from build123d import *

# Parameters (mm, degrees)
PAD010_DEPTH = 31
FILLET004_R  = 1.5
POCKET_DEPTH = 32


with BuildPart() as part:
    # Sketch002 → Pad010 (new body)
    with BuildSketch(Plane.XY):
        Polygon((0, 65), (18, 53), (-18, 53), align=None)
    extrude(amount=PAD010_DEPTH)

    # Fillet004
    fillet004_edges = [part.edges().sort_by_distance(p)[0] for p in [
        (-18, 53, 15.5),
        (18, 53, 15.5),
        (0, 65, 15.5),
        (0, 53, 31),
        (-9, 59, 31),
        (9, 59, 31),
    ]]
    fillet(fillet004_edges, radius=FILLET004_R)

    # Sketch004 (on Face11 of Fillet004) → Pocket (cut)
    with BuildSketch(Plane.XY.offset(31)):
        with BuildLine():
            Line((-11.9466006322, 55.2328239407), (-0.4437599322, 62.9013844075))
            ThreePointArc((0.4437600752, 62.9013843122), (8.59e-08, 63.0357440221), (-0.4437599322, 62.9013844075))
            Line((0.4437600752, 62.9013843122), (11.9466006329, 55.2328239403))
            ThreePointArc((11.724725846, 54.5), (12.1075640333, 54.7840894266), (11.9466006329, 55.2328239403))
            Line((-11.7247263937, 54.5), (11.724725846, 54.5))
            ThreePointArc((-11.9466006322, 55.2328239407), (-12.1075641128, 54.7840896892), (-11.7247263937, 54.5))
        make_face()
    extrude(amount=-POCKET_DEPTH, mode=Mode.SUBTRACT)


solid = part.part
CAD build for the part. Positions are in the model's coordinates, mm. A direction names the side the tool comes from. Round coordinates to 2 decimals unless told otherwise and drop trailing zeros. Loops run counter-clockwise (first coordinate to the right, second up) from the corner with the lowest first, then second, coordinate; pieces in that order, holes last.
(1) Drop a flat-ended pin along its axis: pin 1 (2 mm diameter, centred on y = 60.5, z = 18.5, fed in from +X). Give the stop position or say it passes through.
(2) Cut at A-A (z = 5). Give the cut face in (x, y).
(3) Wall check: line 1 along X through (y, z) = (56.5, 28); line 2 along X through (y, z) = (55, 6); line 3 along Y through (x, z) = (4.5, 13). Give the ranges that are in metal, low to high.
(4) Which spindle directions (+Z, -Z, +X, -X, +Y, -Y) get a long thin tool onto all of the face, cutting with end or side? Do faces 1 (the cylindrical face through (14.49, 54.09, 14.96)), 2 (the flat face through (0, 54.5, 16)). Say none if no direction does.
(5) Two-plate mould, pull along Y, no slides. Class faces 3 (the flat face through (-6.28, 59.01, 15.72)), 4 (the flat face through (7.26, 60.16, 14.54)), 5 (the cylindrical face through (-14.473, 54.04, 14.956)), 6 (the cylindrical face through (0.007, 63.036, 15.717)): +Y half, -Y half, draft (parallel to the pull), parting line (faces both ways), or undercut.
Findings below:
1. pin 1: stops at x = 8.25
2. outline: (-13.88, 55.75) arc R1.5 ccw to (-13.05, 53) - (13.05, 53) arc R1.5 ccw to (13.88, 55.75) - (0.83, 64.45) arc R1.5 ccw to (-0.83, 64.45) - close; hole (-11.95, 55.23) arc R0.4 ccw to (-11.72, 54.5) - (11.72, 54.5) arc R0.4 ccw to (11.95, 55.23) - (0.44, 62.9) arc R0.8 ccw to (-0.44, 62.9) - close
3. line 1: x = -12.75 to -10.05, 10.05 to 12.75
3. line 2: x = -14.46 to -12.11, 12.11 to 14.46
3. line 3: y = 53 to 54.5, 60.2 to 62
4. face 1: +Z, -Z, +X
4. face 2: +Z, -Z
5. face 3: undercut
5. face 4: +Y half
5. face 5: parting line
5. face 6: undercut
